Can you work these out from the model? Positions are in its coordinate system, mm. Face numbers are marked on the shaded views. A direction names the side the tool comes from. Round coordinates to 2 decimals unless told otherwise and drop trailing zeros. Loops run counter-clockwise (first coordinate to the right, second up) from the corner with the lowest first, then second, coordinate; pieces in that order, holes last. Notation, with made-up numbers: (-11, -14.5) - (-4, -14.5) arc R22 ccw to (-4, 12.5) - close; hole circle Ø9 at (59, -31.75). An arc over 180 degrees is marked (long way). Answer as CSV lines item,"result".
```python
from build123d import *

# Parameters (mm, degrees)
RESSALTO_EXTRUS_O1_DEPTH = 10
ESBO_O2_R                = 1.75
CORTE_EXTRUS_O1_DEPTH    = 10


with BuildPart() as part:
    # Esboço1 → Ressalto-extrusão1 (new body)
    with BuildSketch(Plane.XY):
        Polygon((-12, 5), (-22, 5), (-22, 3), (-12, 3), (-12, -15), (12, -15), (12, 3), (22, 3), (22, 5), (12, 5), align=None)
    extrude(amount=RESSALTO_EXTRUS_O1_DEPTH)

    # Esboço2 → Corte-extrusão1 (cut)
    with BuildSketch(Plane(origin=(0, 5, 0), x_dir=(1, 0, 0), z_dir=(0, 1, 0))):
        with Locations(Location((-17.5, -5, 0), (0, 0, 180))):
            Circle(ESBO_O2_R)
        with Locations(Location((17.5, -5, 0), (0, 0, 180))):
            Circle(ESBO_O2_R)
    extrude(amount=-CORTE_EXTRUS_O1_DEPTH, mode=Mode.SUBTRACT)


solid = part.part
```
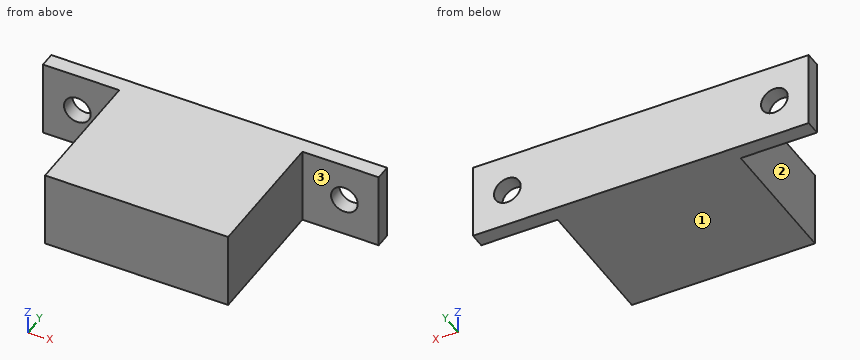
Q1. Imagine slicing it at B-B (z = 5). Write out the boundary of the cut face in (x, y).
Checks:
outline,"(-22, 3) - (-19.25, 3) - (-19.25, 5) - (-22, 5) - close; (-15.75, 3) - (-12, 3) - (-12, -15) - (12, -15) - (12, 3) - (15.75, 3) - (15.75, 5) - (-15.75, 5) - close; (19.25, 3) - (22, 3) - (22, 5) - (19.25, 5) - close"
Q2. On a 3-axis mill with a long thin cutter (end or side, diameter ignored), from which of +Z, -Z, +X, -X, +Y, -Y can I reach the whole of each face in a straight line? I mean the marked faces 1, 2 and 3. Say none if no direction works.
Checks:
face 1,"-Z, +X, -X, +Y, -Y"
face 2,"+Z, -Z, -X, -Y"
face 3,"+Z, -Z, +X, -Y"
Q3. I'm going to push flat-ended pins straight in: pin 1 Ø5.5 at (x, z) = (-17.5, 5) entering from -Y; pin 2 Ø6 at (y, z) = (-12, 2.5) entering from -X; pin 3 Ø3 at (y, z) = (-5, 1.5) entering from +X. Where does each tip first touch, or does it pass through?
Checks:
pin 1,"y = 3"
pin 2,"x = -12"
pin 3,"x = 12"
Q4. Imagine slicing it at D-D (y = -12). Write out the boundary of the cut face in (x, z), then the cut area to 3 significant figures.
Checks:
outline,"(-12, 0) - (12, 0) - (12, 10) - (-12, 10) - close"
area,"240 mm²"
Q5. If I drill on line 1 along Z through (x, y) = (17.5, 4.2); line 2 along Y through (x, z) = (-20, 4.75); line 3 along X through (y, z) = (-7.5, 6.75), over which ranges is the centre line in solid material (lowest first)? Write a range as [from, to].
Checks:
line 1,"[0, 3.25], [6.75, 10]"
line 2,"[3, 5]"
line 3,"[-12, 12]"
Q6. Imagine slicing it at C-C (z = 7.5). Write out the boundary of the cut face in (x, y).
Checks:
outline,"(-22, 3) - (-12, 3) - (-12, -15) - (12, -15) - (12, 3) - (22, 3) - (22, 5) - (-22, 5) - close"
Q7. Imagine slicing it at A-A (x = 17.5). Write out the boundary of the cut face in (y, z), then the cut area to 3 significant figures.
Checks:
outline,"(3, 0) - (5, 0) - (5, 3.25) - (3, 3.25) - close; (3, 6.75) - (5, 6.75) - (5, 10) - (3, 10) - close"
area,"13.0 mm²"
